Model file for the job. Use its own axes, mm. A direction names the side the tool comes from. Round coordinates to 2 decimals unless told otherwise and drop trailing zeros. Write each loop counter-clockwise with the first axis right and the second up, starting at its lowest first coordinate (ties: lowest second). Pieces come first, ordered by that corner, then holes.
```python
from build123d import *

# Parameters (mm, degrees)
SKETCH_R        = 20
PAD_DEPTH       = 20
SKETCH001_R     = 4.5
POCKET_DEPTH    = 1
FILLET_R        = 5
FILLET001_R     = 2
SKETCH002_W     = 5
SKETCH002_H     = 1.5
POCKET001_DEPTH = 1


with BuildPart() as part:
    # Sketch → Pad (new body)
    with BuildSketch(Plane.XY):
        Circle(SKETCH_R)
    extrude(amount=PAD_DEPTH)

    # Sketch001 → Pocket (cut)
    with BuildSketch(Plane.XY):
        Circle(SKETCH001_R)
    extrude(amount=POCKET_DEPTH, mode=Mode.SUBTRACT)

    # Fillet
    fillet_edges = [part.edges().sort_by_distance(p)[0] for p in [
        (-20, 0, 20),
    ]]
    fillet(fillet_edges, radius=FILLET_R)

    # Fillet001
    fillet001_edges = [part.edges().sort_by_distance(p)[0] for p in [
        (-20, 0, 0),
    ]]
    fillet(fillet001_edges, radius=FILLET001_R)

    # Sketch002 → Pocket001 (cut)
    with BuildSketch(Plane.XY.offset(20)):
        with Locations((10.5, 0)):
            Rectangle(SKETCH002_W, SKETCH002_H)
    extrude(amount=-POCKET001_DEPTH, mode=Mode.SUBTRACT)


solid = part.part
```
1) Cut at A-A on y = 0. List the corners of the cut face in (x, z).
2) Cut at C-C on z = 14. List the corners of the cut face in (x, y).
3) Pull direction X, two halves, no side cores. Call faces 4 (the face through (-4.336, -19.524, 8.409)), 5 (the face through (13, 0, 19.5)), 6 (the face through (0, 0, 20)): released by +X, released by -X, zero draft, split by the parting line, or undercut.
4) Which spindle directions (+Z, -Z, +X, -X, +Y, -Y) get a long thin tool onto all of the face, cutting with end or side? Do faces 1 (the face through (4, -4, 0)), 2 (the face through (10.5, -0.75, 19.5)), 3 (the face through (-0.59, 4.46, 0.49)). Say none if no direction does.
5) Cut at B-B on x = 0. List the corners of the cut face in (y, z).
6) Wall check: probe 1 along Z at (x, y) = (16, -9); probe 2 along Y at (x, z) = (-5, 10.5); probe 3 along Y at (x, z) = (18, 11.25). Give the ranges that are in metal, low to high.
7) Flat gauge pins, fed straight in: pin 1 Ø4 at (y, z) = (1.5, 13) entering from -X; pin 2 Ø3 at (x, z) = (-13.5, 14.5) entering from +Y; pin 3 Ø1.2 at (x, y) = (11, 0) entering from +Z; pin 4 Ø1 at (x, z) = (11, 7) entering from -Y. Where does each tip first touch, or does it go through?
Result sheet:
1. outline: (-20, 2) arc R2 ccw to (-18, 0) - (-4.5, 0) - (-4.5, 1) - (4.5, 1) - (4.5, 0) - (18, 0) arc R2 ccw to (20, 2) - (20, 15) arc R5 ccw to (15, 20) - (13, 20) - (13, 19) - (8, 19) - (8, 20) - (-15, 20) arc R5 ccw to (-20, 15) - close
2. outline: circle Ø40 at (0, 0)
3. face 4: split by the parting line
3. face 5: undercut
3. face 6: zero draft
4. face 1: -Z, +X, -X, +Y, -Y
4. face 2: +Z
4. face 3: -Z
5. outline: (-20, 2) arc R2 ccw to (-18, 0) - (-4.5, 0) - (-4.5, 1) - (4.5, 1) - (4.5, 0) - (18, 0) arc R2 ccw to (20, 2) - (20, 15) arc R5 ccw to (15, 20) - (-15, 20) arc R5 ccw to (-20, 15) - close
6. probe 1: z = 0.03 to 18.7
6. probe 2: y = -19.36 to 19.36
6. probe 3: y = -8.72 to 8.72
7. pin 1: stops at x = -20
7. pin 2: stops at y = 16
7. pin 3: stops at z = 19
7. pin 4: stops at y = -17.02
